Can you work these out from the model? Positions are in its coordinate system, mm. A direction names the side the tool comes from. Coordinates: 2 decimals unless noted, no trailing zeros. Order: outer loops, then holes, each group sorted by start corner. A loop starts at its lowest first (then second) coordinate and runs counter-clockwise, first axis right, second up. Notation, with made-up numbers: M 20.5,84.5 L 59.5,84.5 A27 cw 59.5,113.5 Z; hole C -1.75,-28.75 d1. An arc over 180 degrees is marked long. Answer as a JSON object with one key per item and string values.
from build123d import *

# Parameters (mm, degrees)
SKETCH1_R           = 2.1
BOSS_EXTRUDE1_DEPTH = 215
FILLET1_R           = 0.5
CUT_EXTRUDE6_DEPTH  = 3.5
SKETCH11_R          = 4.05
CUT_EXTRUDE7_DEPTH  = 0.5
CUT_EXTRUDE8_DEPTH  = 216


with BuildPart() as part:
    # Sketch1 → Boss-Extrude1 (new body)
    with BuildSketch(Plane(origin=(0, 0, 0), x_dir=(0, 0, -1), z_dir=(1, 0, 0))):
        with BuildLine():
            Line((8, 0), (8, 4.953035538))
            ThreePointArc((8, 4.953035538), (7.10478138, 7.090766893), (4.953403104, 7.952673638))
            Line((4.953403104, 7.952673638), (-5.046596896, 7.797331911))
            ThreePointArc((-5.046596896, 7.797331911), (-7.137731355, 6.902475191), (-8, 4.797693812))
            Line((-8, 4.797693812), (-8, 0))
            ThreePointArc((-8, 0), (0, -8), (8, 0))
        make_face()
        Polygon((-4.098983019, -0.040884468), (-2.014084522, -3.570265658), (2.084898497, -3.529381191), (4.098983019, 0.040884468), (2.014084522, 3.570265658), (-2.084898497, 3.529381191), align=None, mode=Mode.SUBTRACT)
        Polygon((-2.084898497, 3.529381191), (-4.098983019, -0.040884468), (-2.014084522, -3.570265658), (2.084898497, -3.529381191), (4.098983019, 0.040884468), (2.014084522, 3.570265658), align=None)
        Circle(SKETCH1_R, mode=Mode.SUBTRACT)
    extrude(amount=BOSS_EXTRUDE1_DEPTH)

    # Fillet1
    fillet1_edges = [part.edges().sort_by_distance(p)[0] for p in [
        (0, 6.902475191, 7.137731355),
        (0, 7.875002775, 0.046596896),
        (215, 7.090766893, -7.10478138),
        (0, 7.090766893, -7.10478138),
        (0, 2.476517769, -8),
        (215, 7.875002775, 0.046596896),
        (215, 6.902475191, 7.137731355),
        (215, 2.398846906, 8),
        (215, -8, 0),
        (215, 2.476517769, -8),
        (0, -8, 0),
        (0, 2.398846906, 8),
    ]]
    fillet(fillet1_edges, radius=FILLET1_R)

    # Sketch8 → Cut-Extrude6 (cut)
    with BuildSketch(Plane(origin=(209, 0, 0), x_dir=(0, 0, -1), z_dir=(1, 0, 0))):
        Polygon((2.040874515, 3.555019627), (10.204569272, 3.555019627), (10.291698633, -3.544958989), (2.058300051, -3.544958989), (-2.040874515, -3.555019627), (-4.099174565, -0.010060638), (-2.058300051, 3.544958989), align=None)
    cut_extrude6 = extrude(amount=-CUT_EXTRUDE6_DEPTH, mode=Mode.SUBTRACT)

    # Sketch11 → Cut-Extrude7 (cut)
    with BuildSketch(Plane(origin=(215, 0, 0), x_dir=(0, 0, -1), z_dir=(1, 0, 0))):
        Circle(SKETCH11_R)
    cut_extrude7 = extrude(amount=-CUT_EXTRUDE7_DEPTH, mode=Mode.SUBTRACT)

    # Mirror1: Cut-Extrude6, Cut-Extrude7 across plane
    add(cut_extrude6.mirror(Plane.ZY.offset(-107.5)), mode=Mode.SUBTRACT)
    add(cut_extrude7.mirror(Plane.ZY.offset(-107.5)), mode=Mode.SUBTRACT)

    # Sketch13 → Cut-Extrude8 (cut, through all)
    with BuildSketch(Plane.ZY):
        with BuildLine():
            Line((-8.155806574, 4), (-8.155806574, 8.298439356))
            Line((-8.155806574, 8.298439356), (-4.156962159, 8.096142326))
            ThreePointArc((-4.156962159, 8.096142326), (-5.293589836, 5.205771064), (-8.155806574, 4))
        make_face()
    extrude(amount=-CUT_EXTRUDE8_DEPTH, mode=Mode.SUBTRACT)


solid = part.part
Item 1: I want a section at A-A, the plane x = 64.5. Write out the boundary of the cut face in (y, z).
Answers follow:
{"outline": "M 0,-8 L 4,-8 A4 cw 7.94,-4.16 L 7.8,5.05 A3 ccw 4.8,8 L 0,8 A8 ccw Z; hole C 0,0 d4.2"}
Item 2: If we mould it in two halves opening along X, with no side actions, what happens to faces 1 (the flat face through (0.5, -2, -2)), 2 (the flat face through (215, 3, 3)), 3 (the flat face through (106, 2, 8)), 4 (the flat face through (207, -3.545, -5))? For each: pulls with the +X half, pulls with the -X half, needs draft (parallel to the pull), parting line crosses it, or undercut.
Answers follow:
{"face 1": "pulls with the -X half", "face 2": "pulls with the +X half", "face 3": "needs draft", "face 4": "undercut"}
Item 3: Which directions (+Z, -Z, +X, -X, +Y, -Y) give clear straight access to the entire face, cutting with the end or side of a thin tool? Please do faces 5 (the cylindrical face through (106.128, 0.631, -2.003)), 6 (the flat face through (106, 2, -8)), 7 (the cylindrical face through (0.246, -3.954, 0.878)), 8 (the flat face through (205.5, 0, -3)), 9 (the flat face through (214.5, -2, -2)).
Answers follow:
{"face 5": "+X, -X", "face 6": "-Z, +X, -X, +Y, -Y", "face 7": "-X", "face 8": "-Z", "face 9": "+X"}
Item 4: I'm going to push flat-ended pins straight in: pin 1 (2 mm diameter, centred on x = 29.5, y = 6, fed in from -Z); pin 2 (2 mm diameter, centred on x = 152, y = -3.5, fed in from +Z); pin 3 (3 mm diameter, centred on x = 208, z = -6, fed in from -Y). Where does each tip first touch, or does it pass through?
Answers follow:
{"pin 1": "stops at z = -5.51", "pin 2": "stops at z = 7.6", "pin 3": "stops at y = -6.61"}
Item 5: Please list where these lines run through material, in increasing order: line 1 (X direction, y = 0, z = -7.5); line 2 (X direction, y = -0.5, z = 3.25); line 3 (Z direction, x = 211.1, y = 0).
Answers follow:
{"line 1": "x = 0 to 6, 9.5 to 205.5, 209 to 215", "line 2": "x = 0.5 to 6, 9.5 to 205.5, 209 to 214.5", "line 3": "z = -8 to -2.1, 2.1 to 8"}
